The listing builds one solid part. Answer for the finished solid, in the listing's coordinates (mm). A direction names the side the tool comes from. Round coordinates to 2 decimals unless told otherwise and drop trailing zeros. Write each loop counter-clockwise with the first axis right and the second up, starting at its lowest first coordinate (ties: lowest second). Pieces come first, ordered by that corner, then holes. Notation, with made-up numbers: (8.5, 38.5) - (54.5, 38.5) arc R29 cw to (54.5, 63.5) - close; hole circle Ø3 at (70.25, 32.5). An arc over 180 degrees is marked (long way). Return JSON: item names as keys, results as strings. Group by question number.
(1) Which of the six approach directions +Z, -Z, +X, -X, +Y, -Y give full straight-line access (tool end or side, diameter ignored) to faces 1 (the flat face through (2, -91, -61.622)), 2 (the flat face through (1, -100, -49)), 3 (the flat face through (2, -20, -52)), 4 (the cylindrical face through (1.5, -11.9, -35.3)), 5 (the flat face through (2, -91, -36.622))?
(2) Each of these flat-tipped pins is pushed along its axis until it touches: pin 1 (2.5 mm diameter, centred on y = -59, z = -36.875, fed in from +X) (3 decimals); pin 2 (1 mm diameter, centred on x = 0.5, y = -56.5, fed in from +Z); pin 3 (4 mm diameter, centred on y = -42, z = -34, fed in from -X); pin 4 (0.9 mm diameter, centred on x = 1.5, y = -86.5, fed in from +Z). Where does it stop, or does it pass through?
(3) Section B-B, the plane x = 2.55 is taken. Write down the section's boundary in (y, z) (3 decimals).
(4) Find the intervals of material crossed by line 1 along Y through (x, z) = (2.45, -60.5); line 2 along Z through (x, y) = (1.45, -83); line 3 along Z through (x, y) = (1.4, -89.5), in increasing order. Write a range as [from, to].
(5) Determine the mould class of faces 6 (the cylindrical face through (1.479, -78.669, -61.224)), 7 (the cylindrical face through (1.521, -11.575, -61.886)), 8 (the flat face through (3, -38, -29)) for opening direction Z: +Z half, -Z half, draft (parallel to the pull), parting line (faces both ways), or undercut.
(6) Section D-D, the plane z = -25 is taken. Write down the section's boundary in (x, y).
(7) Section A-A, the plane z = -46 is taken. Write down the section's boundary in (x, y).
(8) Section C-C, the plane y = -59 is taken. Write down the section's boundary in (x, z) (3 decimals), then the cut area to 3 significant figures.
```python
from build123d import *

# Parameters (mm, degrees)
CROQUIS1_W              = 75
CROQUIS1_H              = 100
SALIENTE_EXTRUIR1_DEPTH = 3
CORTAR_EXTRUIR1_DEPTH   = 3
REDONDEO1_R             = 10
REDONDEO3_R             = 5
CROQUIS3_R              = 1.5
CORTAR_EXTRUIR2_DEPTH   = 3


with BuildPart() as part:
    # Croquis1 → Saliente-Extruir1 (new body)
    with BuildSketch(Plane(origin=(0, 0, 0), x_dir=(0, 0, -1), z_dir=(1, 0, 0))):
        with Locations((37.5, -50)):
            Rectangle(CROQUIS1_W, CROQUIS1_H)
    extrude(amount=SALIENTE_EXTRUIR1_DEPTH)

    # Croquis2 → Cortar-Extruir1 (cut)
    with BuildSketch(Plane(origin=(3, 0, 0), x_dir=(0, 0, -1), z_dir=(1, 0, 0))):
        Polygon((75, -20), (25, -20), (61.621978753, -78.595166005), (61.621978753, -100), (75, -100), align=None)
        Polygon((0, -100), (36.621978753, -100), (36.621978753, -78.595166005), (0, -20), align=None)
    extrude(amount=-CORTAR_EXTRUIR1_DEPTH, mode=Mode.SUBTRACT)

    # Redondeo1
    redondeo1_edges = [part.edges().sort_by_distance(p)[0] for p in [
        (1.5, -78.595166005, -61.621978753),
        (1.5, -20, 0),
        (1.5, -78.595166005, -36.621978753),
        (1.5, 0, 0),
    ]]
    fillet(redondeo1_edges, radius=REDONDEO1_R)

    # Redondeo3
    redondeo3_edges = [part.edges().sort_by_distance(p)[0] for p in [
        (1.5, -20, -25),
        (1.5, -20, -75),
        (1.5, 0, -75),
    ]]
    fillet(redondeo3_edges, radius=REDONDEO3_R)

    # Croquis3 → Cortar-Extruir2 (cut)
    with BuildSketch(Plane(origin=(3, 0, 0), x_dir=(0, 0, -1), z_dir=(1, 0, 0))):
        with Locations((12.5, -11)):
            Circle(CROQUIS3_R)
        with Locations((12.5, -83)):
            Circle(CROQUIS3_R)
        with Locations((36.5, -11)):
            Circle(CROQUIS3_R)
        with Locations((60.5, -11)):
            Circle(CROQUIS3_R)
        with Locations((21.875, -35)):
            Circle(CROQUIS3_R)
        with Locations((36.875, -59)):
            Circle(CROQUIS3_R)
        with Locations((49.121978753, -83)):
            Circle(CROQUIS3_R)
    extrude(amount=-CORTAR_EXTRUIR2_DEPTH, mode=Mode.SUBTRACT)


solid = part.part
```
Working result:
{
 "1": {"face 1": "-Z, +X, -X, -Y", "face 2": "+Z, -Z, +X, -X, -Y", "face 3": "-Z, +X, -X", "face 4": "+X, -X", "face 5": "+Z, +X, -X, -Y"},
 "2": {"pin 1": "passes through", "pin 2": "stops at z = -22.5", "pin 3": "stops at x = 0", "pin 4": "stops at z = -36.62"},
 "3": {"outline": "(-100, -61.622) - (-81.463, -61.622) arc R10 ccw to (-76.163, -60.102) - (-27.65, -29.781) arc R5 cw to (-20, -34.021) - (-20, -70) arc R5 ccw to (-15, -75) - (-5, -75) arc R5 ccw to (0, -70) - (0, -10) arc R10 ccw to (-10, 0) - (-17.132, 0) arc R10 ccw to (-22.432, -1.52) - (-76.163, -35.102) arc R10 cw to (-81.463, -36.622) - (-100, -36.622) - close; hole circle Ø3 at (-83, -49.122); hole circle Ø3 at (-59, -36.875); hole circle Ø3 at (-35, -21.875); hole circle Ø3 at (-11, -60.5); hole circle Ø3 at (-11, -36.5); hole circle Ø3 at (-11, -12.5)"},
 "4": {"line 1": "y = [-100, -76.86], [-20, -12.5], [-9.5, 0]", "line 2": "z = [-61.62, -50.62], [-47.62, -36.62]", "line 3": "z = [-61.62, -36.62]"},
 "5": {"face 6": "-Z half", "face 7": "undercut", "face 8": "draft"},
 "6": {"outline": "(0, -60) - (3, -60) - (3, 0) - (0, 0) - close"},
 "7": {"outline": "(0, -100) - (3, -100) - (3, -53.6) - (0, -53.6) - close; (0, -20) - (3, -20) - (3, 0) - (0, 0) - close"},
 "8": {"outline": "(0, -49.375) - (3, -49.375) - (3, -38.375) - (0, -38.375) - close; (0, -35.375) - (3, -35.375) - (3, -24.375) - (0, -24.375) - close", "area": "66.0 mm^2"}
}
